Could you check a few things on this drawing? It's one solid part, dimensions in mm from its lowest x, y, z. A direction names the side the tool comes from. Give positions to 0.01 mm unless a question says otherwise; leave off trailing zeros. Order: outer loops, then holes, each group sorted by start corner. A loop starts at its lowest first (then second) coordinate and runs counter-clockwise, first axis right, second up.
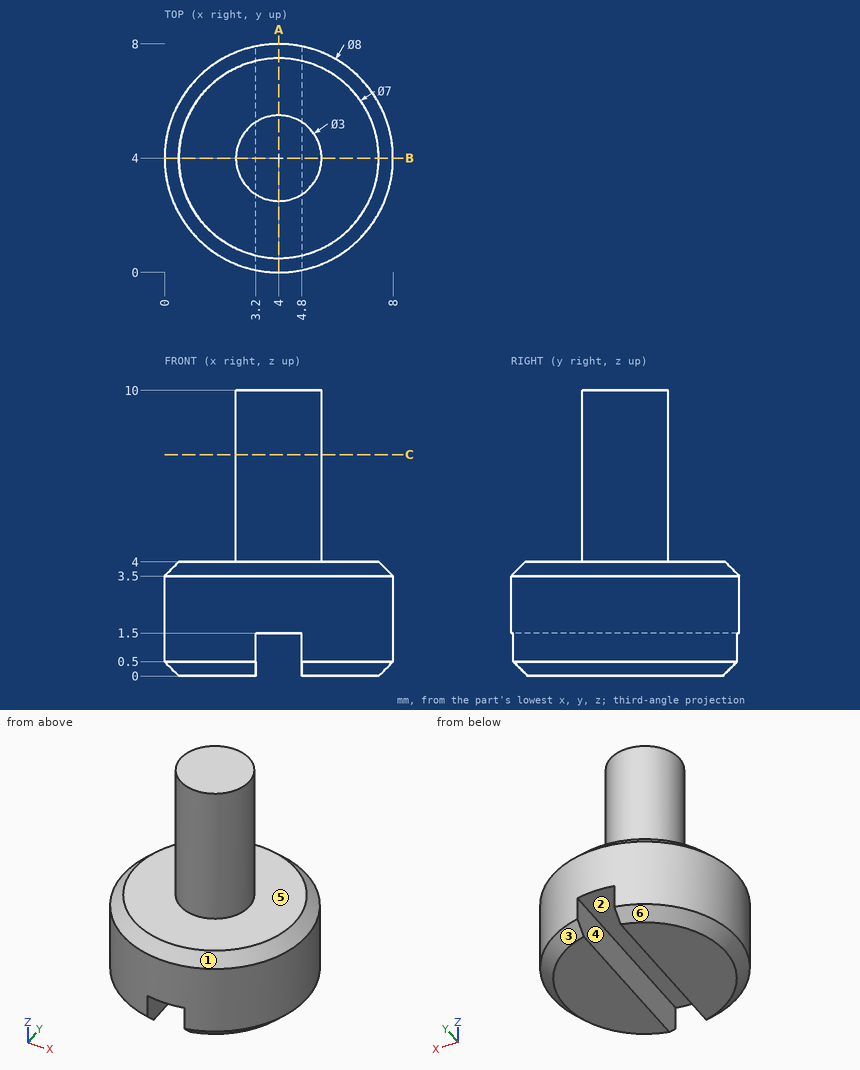
1) Which directions (+Z, -Z, +X, -X, +Y, -Y) give clear straight access to the entire face, cutting with the end or side of a thin tool? Please do the marked faces 5 and 6.
2) I'm going to push flat-ended pins straight in: pin 1 Ø1 at (y, z) = (3.5, 7) entering from -X; pin 2 Ø0.5 at (y, z) = (5.5, 1) entering from +X; pin 3 Ø2 at (y, z) = (3.5, 8.5) entering from +X; pin 4 Ø1.3 at (x, y) = (3.5, 5.5) entering from -Z. Where does each tip first touch, or does it pass through?
3) We'd pull the mould along X, two halves only. Please class the marked faces 1, 2, 3 and 4: +X half, -X half, draft (parallel to the pull), parting line (faces both ways), or undercut.
4) If I drill on line 1 (Z direction, x = 5.75, y = 4.5); line 2 (X direction, y = 4, z = 9.25); line 3 (Z direction, x = 3.5, y = 1.75), over which ranges is the centre line in solid material (lowest first)?
5) Suppose I cut it at B-B (y = 4). Please give me the cut outline in (x, z).
6) Suppose I cut it at A-A (x = 4). Please give me the cut outline in (y, z).
7) Suppose I cut it at C-C (z = 7.75). Please give me the cut outline in (x, y), and give its area (3 significant figures).
Results:
1. face 5: +Z
1. face 6: -Z, -X
2. pin 1: stops at x = 2.5
2. pin 2: stops at x = 7.8
2. pin 3: stops at x = 5.5
2. pin 4: stops at z = 0
3. face 1: parting line
3. face 2: undercut
3. face 3: +X half
3. face 4: undercut
4. line 1: z = 0 to 4
4. line 2: x = 2.5 to 5.5
4. line 3: z = 1.5 to 4
5. outline: (0, 0.5) - (0.5, 0) - (3.2, 0) - (3.2, 1.5) - (4.8, 1.5) - (4.8, 0) - (7.5, 0) - (8, 0.5) - (8, 3.5) - (7.5, 4) - (5.5, 4) - (5.5, 10) - (2.5, 10) - (2.5, 4) - (0.5, 4) - (0, 3.5) - close
6. outline: (0, 1.5) - (8, 1.5) - (8, 3.5) - (7.5, 4) - (5.5, 4) - (5.5, 10) - (2.5, 10) - (2.5, 4) - (0.5, 4) - (0, 3.5) - close
7. outline: circle Ø3 at (4, 4)
7. area: 7.07 mm2
